The model under review builds one solid part; all positions refer to its coordinate system, in mm. Round coordinates to 2 decimals unless told otherwise and drop trailing zeros. Write each loop counter-clockwise with the first axis right and the second up, starting at its lowest first coordinate (ties: lowest second). Pieces come first, ordered by that corner, then holes. Notation, with made-up numbers: (-34, 31) - (-10, 31) arc R20 cw to (-10, 42) - close; hole circle Ø6 at (89.25, 51.5). An arc over 180 degrees is marked (long way). Use one line per item in the form item = value.
from build123d import *

# Parameters (mm, degrees)
SKETCH_1_W      = 50
SKETCH_1_H      = 90
EXTRUDE_1_DEPTH = 130
EXTRUDE_2_DEPTH = 10


with BuildPart() as part:
    # Эскиз1 → Бобышка-Вытянуть1 (new body)
    with BuildSketch(Plane(origin=(0, 0, 0), x_dir=(0, 0, -1), z_dir=(1, 0, 0))):
        with Locations((25, 45)):
            Rectangle(SKETCH_1_W, SKETCH_1_H)
    extrude(amount=-EXTRUDE_1_DEPTH)

    # Эскиз2 → Бобышка-Вытянуть2 (add)
    with BuildSketch(Plane.XY):
        with BuildLine():
            Line((-14, 38), (-14, 52))
            ThreePointArc((-14, 52), (-10, 56), (-6, 52))
            Line((-6, 52), (-6, 38))
            ThreePointArc((-6, 38), (-10, 34), (-14, 38))
        make_face()
    extrude(amount=EXTRUDE_2_DEPTH)


solid = part.part
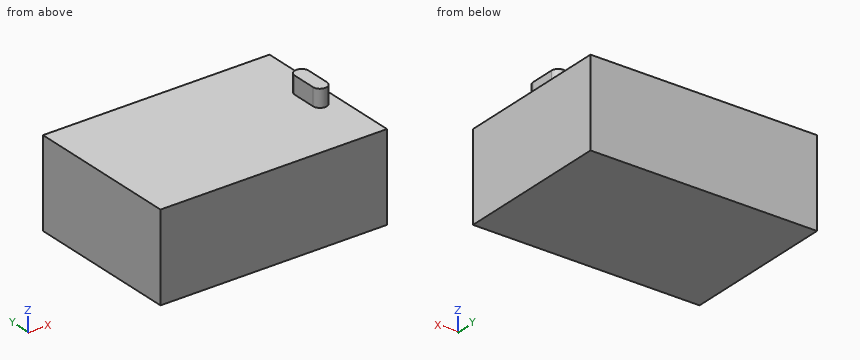
(1) Add section D-D on y = 28.5. Write out the cut boundary in (x, z).
Geometry results:
outline = (-130, -50) - (0, -50) - (0, 0) - (-130, 0) - close
(2) Add section A-A on x = -10. Write out the cut boundary in (y, z), then the cut area to 3 significant figures.
Geometry results:
outline = (0, -50) - (90, -50) - (90, 0) - (56, 0) - (56, 10) - (34, 10) - (34, 0) - (0, 0) - close
area = 4,720 mm2
(3) Insertion check: P1, Ø11, axis at y = 44, z = 7.5, coming from the +X side; P2, Ø5, axis at y = 46, z = 3.5, coming from the -X side; P3, Ø12, axis at x = -80.5, y = 15.5, coming from the +Z side. Each pin has a flat end and moves straight along its axis. Give the tip position at first contact, or say it passes through.
Geometry results:
P1 = -6
P2 = -14
P3 = 0
(4) Add section C-C on z = 3.5. Write out the cut boundary in (x, y), then the cut area to 3 significant figures.
Geometry results:
outline = (-14, 38) arc R4 ccw to (-6, 38) - (-6, 52) arc R4 ccw to (-14, 52) - close
area = 162 mm2
(5) To check wall thickness, follow L1, parallel to Z at x = -120.5, y = 28. State the ranges of the line that lie inside material, in increasing order.
Geometry results:
L1 = -50 to 0
(6) Add section B-B on y = 45. Write out the cut boundary in (x, z), then the cut area to 3 significant figures.
Geometry results:
outline = (-130, -50) - (0, -50) - (0, 0) - (-6, 0) - (-6, 10) - (-14, 10) - (-14, 0) - (-130, 0) - close
area = 6,580 mm2
